Design review of the part built by this model. Coordinates are the model's own, in mm. A direction names the side the tool comes from. Round coordinates to 2 decimals unless told otherwise and drop trailing zeros. Order: outer loops, then holes, each group sorted by start corner. A loop starts at its lowest first (then second) coordinate and runs counter-clockwise, first axis right, second up. Notation, with made-up numbers: (87, 83.5) - (128, 83.5) arc R20 cw to (128, 91.5) - close; hole circle Ø9 at (57.5, 7.25). An arc over 180 degrees is marked (long way). Use CSV: the item, a comma, the result in double quotes.
from build123d import *

# Parameters (mm, degrees)
SM_BASE_FLANGE_1_DEPTH = 12.5
CUT_EXTRUDE_1_DEPTH    = 257.975679783
CUT_EXTRUDE_2_DEPTH    = 260.384367301
OTHER_START            = -247.5
OTHER_1_DEPTH          = 250


# Read off the part's stored shape, not the designer's step: 断开-边角1
# Sheet-metal steps are written as plain solids
with BuildPart() as part:
    # Sketch 1 → 基体-法兰1 (new, symmetric)
    with BuildSketch(Plane.XY):
        with BuildLine():
            Line((68, 0), (2, 0))
            ThreePointArc((2, 0), (0.585786438, -0.585786438), (0, -2))
            Line((0, -2), (0, -243))
            ThreePointArc((0, -243), (0.585786438, -244.414213562), (2, -245))
            Line((2, -245), (68, -245))
            Line((68, -245), (68, -247.5))
            Line((68, -247.5), (2, -247.5))
            ThreePointArc((2, -247.5), (-1.181980515, -246.181980515), (-2.5, -243))
            Line((-2.5, -243), (-2.5, -2))
            ThreePointArc((-2.5, -2), (-1.181980515, 1.181980515), (2, 2.5))
            Line((2, 2.5), (68, 2.5))
            Line((68, 2.5), (68, 0))
        make_face()
    extrude(amount=SM_BASE_FLANGE_1_DEPTH, both=True)

    # 草图4 → 切除-拉伸1 (cut, through all)
    with BuildSketch(Plane(origin=(0, 0, 0), x_dir=(0, 0, -1), z_dir=(1, 0, 0))):
        with BuildLine():
            Line((2.5, -22.5), (2.5, -27.5))
            ThreePointArc((2.5, -27.5), (0, -30), (-2.5, -27.5))
            Line((-2.5, -27.5), (-2.5, -22.5))
            ThreePointArc((-2.5, -22.5), (0, -20), (2.5, -22.5))
        make_face()
        with BuildLine():
            Line((2.5, -112.5), (2.5, -117.5))
            ThreePointArc((2.5, -117.5), (0, -120), (-2.5, -117.5))
            Line((-2.5, -117.5), (-2.5, -112.5))
            ThreePointArc((-2.5, -112.5), (0, -110), (2.5, -112.5))
        make_face()
        with BuildLine():
            Line((2.5, -207.5), (2.5, -202.5))
            ThreePointArc((2.5, -202.5), (0, -200), (-2.5, -202.5))
            Line((-2.5, -202.5), (-2.5, -207.5))
            ThreePointArc((-2.5, -207.5), (0, -210), (2.5, -207.5))
        make_face()
    extrude(amount=-CUT_EXTRUDE_1_DEPTH, mode=Mode.SUBTRACT)

    # 草图7 → 切除-拉伸2 (cut, through all)
    with BuildSketch(Plane(origin=(0, 2.5, 0), x_dir=(1, 0, 0), z_dir=(0, 1, 0))):
        with BuildLine():
            Line((39, 2.5), (61, 2.5))
            ThreePointArc((61, 2.5), (63.5, 0), (61, -2.5))
            Line((61, -2.5), (39, -2.5))
            ThreePointArc((39, -2.5), (36.5, 0), (39, 2.5))
        make_face()
        with BuildLine():
            Line((31, 2.5), (9, 2.5))
            ThreePointArc((9, 2.5), (6.5, 0), (9, -2.5))
            Line((9, -2.5), (31, -2.5))
            ThreePointArc((31, -2.5), (33.5, 0), (31, 2.5))
        make_face()
    extrude(amount=-CUT_EXTRUDE_2_DEPTH, mode=Mode.SUBTRACT)

    # Other 1 outline → Other 1 (cut)
    with BuildSketch(Plane(origin=(0, 0, 0), x_dir=(1, 0, 0), z_dir=(0, 1, 0)).offset(OTHER_START)):
        with BuildLine():
            Line((68, -12.5), (68, -10.5))
            ThreePointArc((68, -10.5), (67.414213562, -11.914213562), (66, -12.5))
            Line((66, -12.5), (68, -12.5))
        make_face()
        with BuildLine():
            ThreePointArc((66, 12.5), (67.414213562, 11.914213562), (68, 10.5))
            Line((68, 10.5), (68, 12.5))
            Line((68, 12.5), (66, 12.5))
        make_face()
    extrude(amount=OTHER_1_DEPTH, mode=Mode.SUBTRACT)


solid = part.part
1) Insertion check: pin 1 Ø12.5 at (y, z) = (-170.5, 3.5) entering from +X. The pin has a flat end and moves straight along its axis. Give the tip position at first contact, or say it passes through.
Data:
pin 1,"stops at x = 0"
2) We need section C-C (y = -182). Give the boundary of the cut face in (x, z).
Data:
outline,"(-2.5, -12.5) - (0, -12.5) - (0, 12.5) - (-2.5, 12.5) - close"
3) For faces 1 (the face through (35, -245, 0)), 2 (the face through (-1.147, -246.217, 0.175)), list the 3-axis set-ups (+Z, -Z, +X, -X, +Y, -Y) from which the entire face can be reached by the end or side of a thin tool; tool diameter is ignored.
Data:
face 1,"+Z, -Z, +X"
face 2,"+Z, -Z, -X, -Y"
4) We need section A-A (x = 20). Give the boundary of the cut face in (y, z).
Data:
outline,"(-247.5, -12.5) - (-245, -12.5) - (-245, -2.5) - (-247.5, -2.5) - close; (-247.5, 2.5) - (-245, 2.5) - (-245, 12.5) - (-247.5, 12.5) - close; (0, -12.5) - (2.5, -12.5) - (2.5, -2.5) - (0, -2.5) - close; (0, 2.5) - (2.5, 2.5) - (2.5, 12.5) - (0, 12.5) - close"
5) To check wall thickness, follow L1, parallel to Y at x = 52.5, z = 9.5; L2, parallel to X at y = -187, z = 6.5. State the ranges of each line that lie inside material, in increasing order. Write a range as from..to.
Data:
L1,"y = -247.5..-245, 0..2.5"
L2,"x = -2.5..0"
6) The part is to be moulded in two halves that separate along Y. For faces 3 (the face through (35, -247.5, 0)), 4 (the face through (35, 0, 0)), 5 (the face through (0, -121, 0)), 6 (the face through (35, 2.5, 0)), say which applies: +Y half, -Y half, draft (parallel to the pull), parting line (faces both ways), or undercut.
Data:
face 3,"-Y half"
face 4,"undercut"
face 5,"undercut"
face 6,"+Y half"
7) We need section B-B (z = -6). Give the boundary of the cut face in (x, y), then the cut area to 3 significant figures.
Data:
outline,"(-2.5, -243) arc R4.5 ccw to (2, -247.5) - (68, -247.5) - (68, -245) - (2, -245) arc R2 cw to (0, -243) - (0, -2) arc R2 cw to (2, 0) - (68, 0) - (68, 2.5) - (2, 2.5) arc R4.5 ccw to (-2.5, -2) - close"
area,"958 mm2"
